```python
from build123d import *

# Parameters (mm, degrees)
CROQUIS1_W              = 200
CROQUIS1_H              = 150.1
SALIENTE_EXTRUIR1_DEPTH = 5
CROQUIS2_R              = 1.5
CROQUIS2_R_2            = 2
CORTAR_EXTRUIR1_DEPTH   = 10
CORTAR_EXTRUIR2_DEPTH   = 400


with BuildPart() as part:
    # Croquis1 → Saliente-Extruir1 (new body)
    with BuildSketch(Plane.XY):
        with Locations((100, 5.648844896)):
            Rectangle(CROQUIS1_W, CROQUIS1_H)
    extrude(amount=SALIENTE_EXTRUIR1_DEPTH)

    # Croquis2 → Cortar-Extruir1 (cut)
    with BuildSketch(Plane.XY.offset(5)):
        with Locations((88, 14.648844896)):
            Circle(CROQUIS2_R)
        with Locations((112, 14.648844896)):
            Circle(CROQUIS2_R)
        with Locations((88, -3.351155104)):
            Circle(CROQUIS2_R)
        with Locations((112, -3.351155104)):
            Circle(CROQUIS2_R)
        with Locations((16, 14.648844896)):
            Circle(CROQUIS2_R_2)
        with Locations((40, 14.648844896)):
            Circle(CROQUIS2_R_2)
        with Locations((40, -3.351155104)):
            Circle(CROQUIS2_R_2)
        with Locations((16, -3.351155104)):
            Circle(CROQUIS2_R_2)
        with Locations((184, -3.351155104)):
            Circle(CROQUIS2_R_2)
        with Locations((160, -3.351155104)):
            Circle(CROQUIS2_R_2)
        with Locations((160, 14.648844896)):
            Circle(CROQUIS2_R_2)
        with Locations((184, 14.648844896)):
            Circle(CROQUIS2_R_2)
    extrude(amount=-CORTAR_EXTRUIR1_DEPTH, mode=Mode.SUBTRACT)

    # Croquis3 → Cortar-Extruir2 (cut)
    with BuildSketch(Plane(origin=(0, 0, 0), x_dir=(-1, 0, 0), z_dir=(0, 0, -1))):
        with BuildLine():
            Line((-195.915748263, 31.98223599), (-157.401555296, 72.845794728))
            ThreePointArc((-157.401555296, 72.845794728), (-149.116372199, 78.651772224), (-139.208641525, 80.698844896))
            Line((-139.208641525, 80.698844896), (-200, 80.698844896))
            Line((-200, 80.698844896), (-200, 21.694066091))
            ThreePointArc((-200, 21.694066091), (-198.941596464, 27.2286743), (-195.915748263, 31.98223599))
        make_face()
        with BuildLine():
            Line((0, 80.698844896), (-60.791358475, 80.698844896))
            ThreePointArc((-60.791358475, 80.698844896), (-50.883627801, 78.651772224), (-42.598444704, 72.845794728))
            Line((-42.598444704, 72.845794728), (-4.084251737, 31.98223599))
            ThreePointArc((-4.084251737, 31.98223599), (-1.058403536, 27.2286743), (0, 21.694066091))
            Line((0, 21.694066091), (0, 80.698844896))
        make_face()
        with BuildLine():
            Line((0, -69.401155104), (0, -10.396376298))
            ThreePointArc((0, -10.396376298), (-1.058403536, -15.930984508), (-4.084251737, -20.684546197))
            Line((-4.084251737, -20.684546197), (-42.598444704, -61.548104935))
            ThreePointArc((-42.598444704, -61.548104935), (-50.883627801, -67.354082431), (-60.791358475, -69.401155104))
            Line((-60.791358475, -69.401155104), (0, -69.401155104))
        make_face()
        with BuildLine():
            ThreePointArc((-195.915748263, -20.684546197), (-198.941596464, -15.930984508), (-200, -10.396376298))
            Line((-200, -10.396376298), (-200, -69.401155104))
            Line((-200, -69.401155104), (-139.208641525, -69.401155104))
            ThreePointArc((-139.208641525, -69.401155104), (-149.116372199, -67.354082431), (-157.401555296, -61.548104935))
            Line((-157.401555296, -61.548104935), (-195.915748263, -20.684546197))
        make_face()
    extrude(amount=-CORTAR_EXTRUIR2_DEPTH, mode=Mode.SUBTRACT)


solid = part.part
```
Input: part model. Units: mm. Frame: model coordinates. Coordinates: 2 decimals unless noted, no trailing zeros. Loops run counter-clockwise (first coordinate to the right, second up) from the corner with the lowest first, then second, coordinate; pieces in that order, holes last. Notation, with made-up numbers: M -36,65.5 L -16,65.5 A15 ccw -16,72.5 Z; hole C -22.5,15.25 d8. An arc over 180 degrees is marked long. Use a Markdown table: item, result. Add a question column.
1) Section B-B, the plane x = 26. Return the cut outline in (y, z).
2) Draft query along X for faces 1 (the flat face through (176.39, -41.4, 2.46)), 2 (the cylindrical face through (1.088, 27.302, 2.465)), 3 (the cylindrical face through (41.847, 13.883, 2.535)). Return one class per face: +X half, -X half, draft (parallel to the pull), parting line (faces both ways), or undercut.
3) Section A-A, the plane z = 4.1. Give the number of separate pieces and of enclosed holes in the cut face, plus the area to 3 significant figures.
4) Section C-C, the plane y = -24. Return the cut outline in (x, z), plus the area to 3 significant figures.
5) Line query: L1, parallel to Y at x = 88, z = 3.65; L2, parallel to Y at x = 184, z = 3.3; L3, parallel to X at y = -11.5, z = 2.7. Output: solid intervals per line, ascending. Write a range as from..to.
6) Pin query (flat end, axial travel): P1, Ø3.5, axis at x = 112, y = 14.65, coming from the +Z side. Return the tip coordinate at first contact, or that it passes through.
Answer below:
| question | item | result |
|---|---|---|
| 1 | outline | M -43.94,0 L 55.23,0 L 55.23,5 L -43.94,5 Z |
| 2 | face 1 | +X half |
| 2 | face 2 | -X half |
| 2 | face 3 | undercut |
| 3 | separate pieces | 1 |
| 3 | enclosed holes | 12 |
| 3 | area | 24,500 mm2 |
| 4 | outline | M 7.21,0 L 192.79,0 L 192.79,5 L 7.21,5 Z |
| 4 | area | 928 mm2 |
| 5 | L1 | -69.4..-4.85, -1.85..13.15, 16.15..80.7 |
| 5 | L2 | -33.33..-5.35, -1.35..12.65, 16.65..44.62 |
| 5 | L3 | 0.04..199.96 |
| 6 | P1 | z = 5 |
